Autodesk Inventor part; units mm, degrees
ref_plane "YZ Plane" through (0, 0, 0) normal (1, 0, 0) x (0, 1, 0)
ref_plane "XZ Plane" through (0, 0, 0) normal (0, 1, 0) x (-1, 0, 0)
ref_plane "XY Plane" through (0, 0, 0) normal (0, 0, 1) x (1, 0, 0)
sketch "Szkic1" plane through (0, 0, 0) normal (0, 0, 1) x (1, 0, 0)
  circle A0 centre (0, 0) radius 8
  dimension "d0" = 16
extrude "Wyciągnięcie proste2" add sketch "Szkic1" along normal blind 1000
sketch "Szkic2" plane through (0, 0, 1000) normal (0, 0, 1) x (1, 0, 0)
  circle A0 centre (0, 0) radius 4
  circle A1 centre (0, 0) radius 8
  dimension "d7" = 8
extrude "Wyciągnięcie proste3" cut sketch "Szkic2" against normal blind 30
sketch "Szkic3" plane through (0, 0, 970) normal (0, 0, 1) x (1, 0, 0)
  circle A0 centre (0, 0) radius 8
  circle A1 centre (0, 0) radius 5
  dimension "d10" = 10
extrude "Wyciągnięcie proste4" cut sketch "Szkic3" against normal blind 30
sketch "Szkic4" plane through (0, 0, 970) normal (0, 0, 1) x (1, 0, 0)
  circle A0 centre (0, 0) radius 5
  circle A1 centre (0, 0) radius 4.98
  dimension "d13" = 9.96
extrude "Wyciągnięcie proste5" cut sketch "Szkic4" against normal blind 20
thread "Gwint2"
sketch "Szkic5" plane through (0, 0, 0) normal (0, 0, -1) x (-1, 0, 0)
  circle A0 centre (0, 0) radius 5
  circle A1 centre (0, 0) radius 8
  dimension "d18" = 10
extrude "Wyciągnięcie proste6" cut sketch "Szkic5" against normal blind 20
thread "Gwint3"
sketch "Szkic6" plane through (0, 0, 940) normal (0, 0, 1) x (1, 0, 0)
  circle A0 centre (0, 0) radius 5
  circle A1 centre (0, 0) radius 8
extrude "Wyciągnięcie proste7" cut sketch "Szkic6" against normal blind 14
sketch "Szkic7" plane through (0, 0, 950) normal (0, 0, 1) x (1, 0, 0)
  circle A0 centre (0, 0) radius 4.98
  circle A1 centre (0, 0) radius 5
extrude "Wyciągnięcie proste8" cut sketch "Szkic7" against normal blind 15
sketch "Szkic8" plane through (0, 0, 970) normal (0, 0, 1) x (1, 0, 0)
  circle A0 centre (0, 0) radius 4.98
  circle A1 centre (0, 0) radius 4
extrude "Wyciągnięcie proste9" cut sketch "Szkic8" against normal blind 15
sketch "Szkic9" plane through (0, 0, 1000) normal (0, 0, 1) x (1, 0, 0)
  circle A0 centre (0, 0) radius 4
extrude "Wyciągnięcie proste10" cut sketch "Szkic9" against normal blind 15.9
properties part number "Śruba trapezowa fi10mm"
The listing builds one solid part. Answer for the finished solid, in the listing's coordinates (mm). A direction names the side the tool comes from. Give positions to 0.01 mm unless a question says otherwise; leave off trailing zeros. Write each loop counter-clockwise with the first axis right and the second up, starting at its lowest first coordinate (ties: lowest second). Pieces come first, ordered by that corner, then holes. Notation, with made-up numbers: M 44.5,1 L 71.5,1 A14 ccw 71.5,15 Z; hole C 76.5,82.5 d9. An arc over 180 degrees is marked long. Write each question's results on one line, items separated by ' | '.
Q1. A tool of negligible diameter and unlimited length cuts with its end or side. For faces 1 (the cylindrical face through (-1.73, 7.81, 466.66)), 2 (the flat face through (-0.1, -5.2, 926)), 3 (the flat face through (0.1, -5.2, 20)), from which of +Z, -Z, +X, -X, +Y, -Y can it reach the whole face along a straight path? Write none if from no direction.
Output values:
face 1: +Z, -Z | face 2: +Z | face 3: -Z
Q2. Flat-ended cylindrical pins translate along their axes: P1, Ø1, axis at x = 4, z = 330, coming from the -Y side; P2, Ø1.5, axis at x = -1.5, z = 277.5, coming from the -Y side; P3, Ø4, axis at y = 4, z = 240, coming from the -X side. Find the tip coordinate at first contact, or state that the pin passes through.
Output values:
P1: y = -7.19 | P2: y = -7.96 | P3: x = -7.75
Q3. Consider L1, parallel to X at y = 1.5, z = 403.5; L2, parallel to Z at x = -1, y = -5.75; L3, parallel to Y at x = 1.25, z = 155. Determine where each line is inside the solid, lowest interval first. Write a range as from..to.
Output values:
L1: -7.86..7.86 | L2: 20..926 | L3: -7.9..7.9
Q4. Section C-C, the plane z = 126 is taken. Write down the section's boundary in (x, y), then the cut area to 3 significant figures.
Output values:
outline: C 0,0 d16 | area: 201 mm2
